Geometry check sheet. Reference: the model listing, model coordinates, mm. Face numbers are marked on the shaded views. Give positions to 0.01 mm unless a question says otherwise; leave off trailing zeros. Write each loop counter-clockwise with the first axis right and the second up, starting at its lowest first coordinate (ties: lowest second). Pieces come first, ordered by that corner, then holes. Notation, with made-up numbers: M 67.25,10 L 111.25,10 A4 ccw 111.25,15 Z; hole C 64,-24.5 d1. An arc over 180 degrees is marked long. Write each question's results on one line, items separated by ' | '.
```python
from build123d import *

# Parameters (mm, degrees)
CROQUIS1_W                = 25.4
CROQUIS1_H                = 25.4
SALIENTE_EXTRUIR1_DEPTH   = 1000
SALIENTE_EXTRUIR1_2_DEPTH = 1000
SALIENTE_EXTRUIR1_3_DEPTH = 1000
SALIENTE_EXTRUIR1_4_DEPTH = 1000
CROQUIS3_W                = 1449.2
CROQUIS3_H                = 25.4
SALIENTE_EXTRUIR2_DEPTH   = 25.4
CROQUIS4_W                = 1449.2
CROQUIS4_H                = 25.4
SALIENTE_EXTRUIR3_DEPTH   = 25.4
CROQUIS5_W                = 1449.2
CROQUIS5_H                = 25.4
SALIENTE_EXTRUIR4_DEPTH   = 25.4
CROQUIS6_W                = 1449.2
CROQUIS6_H                = 25.4
SALIENTE_EXTRUIR5_DEPTH   = 25.4
CROQUIS7_W                = 1500
CROQUIS7_H                = 1500
SALIENTE_EXTRUIR6_DEPTH   = 1.9


with BuildPart() as part:
    # Croquis1 → Saliente-Extruir1 (new body)
    with BuildSketch(Plane(origin=(0, 0, 0), x_dir=(1, 0, 0), z_dir=(0, 1, 0))):
        with Locations((12.7, -12.7)):
            Rectangle(CROQUIS1_W, CROQUIS1_H)
    extrude(amount=SALIENTE_EXTRUIR1_DEPTH)



with BuildPart() as body_2:
    # Croquis1 → Saliente-Extruir1 2 (new body)
    with BuildSketch(Plane(origin=(0, 0, 0), x_dir=(1, 0, 0), z_dir=(0, 1, 0))):
        with Locations((1487.3, -12.7)):
            Rectangle(CROQUIS1_W, CROQUIS1_H)
    extrude(amount=SALIENTE_EXTRUIR1_2_DEPTH)



with BuildPart() as body_3:
    # Croquis1 → Saliente-Extruir1 3 (new body)
    with BuildSketch(Plane(origin=(0, 0, 0), x_dir=(1, 0, 0), z_dir=(0, 1, 0))):
        with Locations((1487.3, -1487.3)):
            Rectangle(CROQUIS1_W, CROQUIS1_H)
    extrude(amount=SALIENTE_EXTRUIR1_3_DEPTH)



with BuildPart() as body_4:
    # Croquis1 → Saliente-Extruir1 4 (new body)
    with BuildSketch(Plane(origin=(0, 0, 0), x_dir=(1, 0, 0), z_dir=(0, 1, 0))):
        with Locations((12.7, -1487.3)):
            Rectangle(CROQUIS1_W, CROQUIS1_H)
    extrude(amount=SALIENTE_EXTRUIR1_4_DEPTH)


with BuildPart() as body_3_1:
    add(body_3.part)

    add(body_4.part)  # Saliente-Extruir2 merges body 4
    # Croquis3 → Saliente-Extruir2 (add)
    with BuildSketch(Plane.XY.offset(1500)):
        with Locations((750, 987.3)):
            Rectangle(CROQUIS3_W, CROQUIS3_H)
        with Locations((750, 561.9)):
            Rectangle(CROQUIS3_W, CROQUIS3_H)
    extrude(amount=-SALIENTE_EXTRUIR2_DEPTH)


with BuildPart() as body_2_1:
    add(body_2.part)

    add(body_3_1.part)  # Saliente-Extruir3 merges body 3
    # Croquis4 → Saliente-Extruir3 (add)
    with BuildSketch(Plane(origin=(1500, 0, 0), x_dir=(0, 0, -1), z_dir=(1, 0, 0))):
        with Locations((-750, 987.3)):
            Rectangle(CROQUIS4_W, CROQUIS4_H)
        with Locations((-750, 561.9)):
            Rectangle(CROQUIS4_W, CROQUIS4_H)
    extrude(amount=-SALIENTE_EXTRUIR3_DEPTH)


with BuildPart() as part_1:
    add(part.part)

    add(body_2_1.part)  # Saliente-Extruir4 merges body 2
    # Croquis5 → Saliente-Extruir4 (add)
    with BuildSketch(Plane(origin=(0, 0, 0), x_dir=(-1, 0, 0), z_dir=(0, 0, -1))):
        with Locations((-750, 987.3)):
            Rectangle(CROQUIS5_W, CROQUIS5_H)
        with Locations((-750, 561.9)):
            Rectangle(CROQUIS5_W, CROQUIS5_H)
    extrude(amount=-SALIENTE_EXTRUIR4_DEPTH)

    # Croquis6 → Saliente-Extruir5 (add)
    with BuildSketch(Plane.ZY):
        with Locations((750, 987.3)):
            Rectangle(CROQUIS6_W, CROQUIS6_H)
        with Locations((750, 561.9)):
            Rectangle(CROQUIS6_W, CROQUIS6_H)
    extrude(amount=-SALIENTE_EXTRUIR5_DEPTH)

    # Croquis7 → Saliente-Extruir6 (add)
    with BuildSketch(Plane(origin=(0, 1000, 0), x_dir=(1, 0, 0), z_dir=(0, 1, 0))):
        with Locations((750, -750)):
            Rectangle(CROQUIS7_W, CROQUIS7_H)
    extrude(amount=SALIENTE_EXTRUIR6_DEPTH)


solid = part_1.part
```
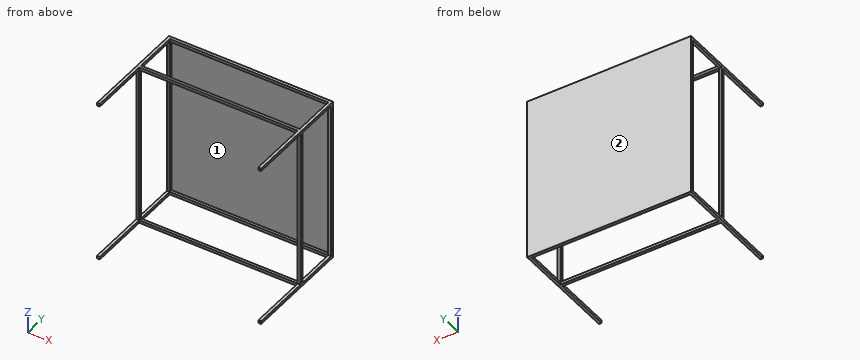
Q1. Section check B-B (x = 1035.5). Enter the section's corners in (y, z).
Answer key:
outline: M 549.2,0 L 574.6,0 L 574.6,25.4 L 549.2,25.4 Z; M 549.2,1474.6 L 574.6,1474.6 L 574.6,1500 L 549.2,1500 Z; M 974.6,0 L 1001.9,0 L 1001.9,1500 L 974.6,1500 L 974.6,1474.6 L 1000,1474.6 L 1000,25.4 L 974.6,25.4 Z
Q2. Depth check by flat-ended pin: P1, Ø20.5, axis at x = 14, z = 662, coming from the -Y side; P2, Ø4, axis at x = 1303.5, z = 650.5, coming from the -Y side. Enter the tip coordinate at first touch or a pass-through.
Answer key:
P1: stops at y = 549.2 | P2: stops at y = 1000
Q3. Section check A-A (z = 894). Enter the section's corners in (x, y), then the cut area to 3 significant figures.
Answer key:
outline: M 0,549.2 L 25.4,549.2 L 25.4,574.6 L 0,574.6 Z; M 0,974.6 L 25.4,974.6 L 25.4,1000 L 1474.6,1000 L 1474.6,974.6 L 1500,974.6 L 1500,1001.9 L 0,1001.9 Z; M 1474.6,549.2 L 1500,549.2 L 1500,574.6 L 1474.6,574.6 Z | area: 5,430 mm2
Q4. Release check for a two-part mould opening along Z. For the marked faces 1 and 2 record: released by +Z, released by -Z, zero draft, split by the parting line, or undercut.
Answer key:
face 1: undercut | face 2: zero draft
Q5. Material ranges on probe 1 along Z at (x, y) = (348.5, 572.5); probe 2 along Y at (x, z) = (73.5, 1066.5), recorded low to high. Write a range as [from, to].
Answer key:
probe 1: z = [0, 25.4], [1474.6, 1500] | probe 2: y = [1000, 1001.9]
Q6. Section check C-C (y = 713.5). Enter the section's corners in (x, z).
Answer key:
outline: M 0,0 L 25.4,0 L 25.4,25.4 L 0,25.4 Z; M 0,1474.6 L 25.4,1474.6 L 25.4,1500 L 0,1500 Z; M 1474.6,0 L 1500,0 L 1500,25.4 L 1474.6,25.4 Z; M 1474.6,1474.6 L 1500,1474.6 L 1500,1500 L 1474.6,1500 Z
